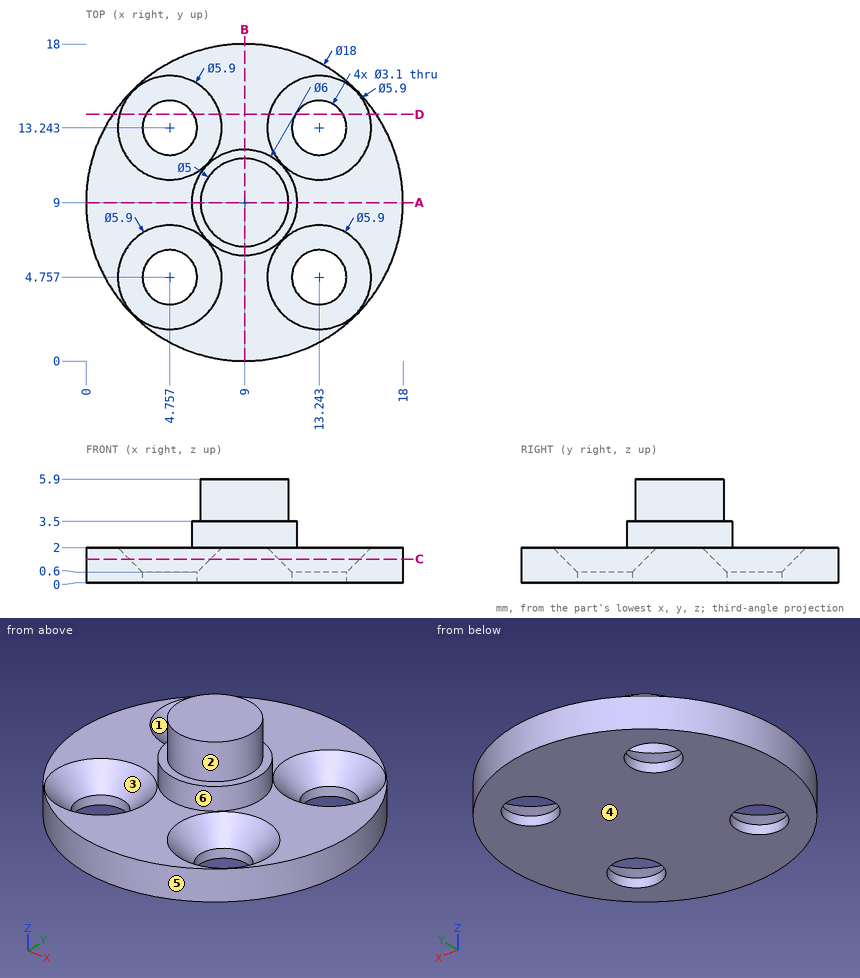
Part print with two shaded views. Sizes in mm from the minimum x, y, z corner. A direction names the side the tool comes from. Coordinates: 2 decimals unless noted, no trailing zeros. Write each loop counter-clockwise with the first axis right and the second up, starting at its lowest first coordinate (ties: lowest second). Pieces come first, ordered by that corner, then holes. Notation, with made-up numbers: M 68.25,2 L 87.25,2 A32 ccw 87.25,33 Z; hole C -30.5,1.25 d9. An arc over 180 degrees is marked long. Return JSON: item names as keys, results as strings.
Item 1: Which spindle directions (+Z, -Z, +X, -X, +Y, -Y) get a long thin tool onto all of the face, cutting with end or side? Do the marked faces 5 and 6. Say none if no direction does.
Findings below:
{"face 5": "+Z, -Z", "face 6": "+Z"}
Item 2: Slice it at A-A, the plane y = 9. Write the cut outline in (x, z), and give its area (3 significant figures).
Findings below:
{"outline": "M 0,0 L 18,0 L 18,2 L 12,2 L 12,3.5 L 11.5,3.5 L 11.5,5.9 L 6.5,5.9 L 6.5,3.5 L 6,3.5 L 6,2 L 0,2 Z", "area": "57.0 mm2"}
Item 3: Slice it at C-C, the plane z = 1.35. Write the cut outline in (x, y).
Findings below:
{"outline": "C 9,9 d18; hole C 4.76,4.76 d4.6; hole C 4.76,13.24 d4.6; hole C 13.24,4.76 d4.6; hole C 13.24,13.24 d4.6"}
Item 4: Drop flat-ended pins along their axis: pin 1 Ø1 at (y, z) = (10, 1.5) entering from +X; pin 2 Ø1.5 at (x, y) = (7.5, 12) entering from +Z; pin 3 Ø6 at (x, y) = (14.5, 14) entering from +Z. Give the stop position or say it passes through.
Findings below:
{"pin 1": "stops at x = 17.99", "pin 2": "stops at z = 3.5", "pin 3": "stops at z = 2"}
Item 5: Probe line 1 (Y direction, x = 14, z = 0.55) (1 decimal); line 2 (Y direction, x = 5.5, z = 0.5); line 3 (Z direction, x = 10.5, y = 1.25). List the from-to ranges inside material, lowest first. Write a range as from..to.
Findings below:
{"line 1": "y = 1.5..3.4, 6.1..11.9, 14.6..16.5", "line 2": "y = 0.71..3.4, 6.12..11.88, 14.6..17.29", "line 3": "z = 0..2"}
Item 6: Two-plate mould, pull along X, no slides. Class the marked faces 1, 2, 3 and 4: +X half, -X half, draft (parallel to the pull), parting line (faces both ways), or undercut.
Findings below:
{"face 1": "undercut", "face 2": "parting line", "face 3": "undercut", "face 4": "draft"}
Item 7: Slice it at D-D, the plane y = 14. State how many separate pieces and enclosed holes the cut face has.
Findings below:
{"separate pieces": "3", "enclosed holes": "0"}
